Read the model definition and answer for the solid it produces. Units are mm, in the model's axes. A direction names the side the tool comes from. Coordinates: 2 decimals unless noted, no trailing zeros. Write each loop counter-clockwise with the first axis right and the second up, starting at its lowest first coordinate (ties: lowest second). Pieces come first, ordered by that corner, then holes. Notation, with made-up numbers: (87, 74) - (128, 74) arc R22 cw to (128, 113) - close; hole circle Ø11 at (-28, 5.5). An arc over 180 degrees is marked (long way). Return JSON: item names as keys, results as strings.
```python
from build123d import *

# Parameters (mm, degrees)
F0_R            = 5
F1_DEPTH        = 50
F2_R            = 15
F3_DEPTH        = 5
F3_COPIES_COUNT = 3
F4_W            = 25
F4_H            = 25
F5_DEPTH        = 5
F5_COPIES_COUNT = 3
F7_DEPTH        = 5
F7_COPIES_COUNT = 3


# Not quite as in the source:
# - a pattern or mirror of a feature is missing from the dataset's text; its kind, count and spacing are read off the source's solid


with BuildPart() as f1:
    # F0 (on Top) → F1 (new body)
    with BuildSketch(Plane.XY):
        Polygon((64.2787609687, 76.6044443119), (0, 100), (-64.2787609687, 76.6044443119), (-98.4807753012, 17.3648177667), (-86.6025403784, -50), (-34.2020143326, -93.9692620786), (34.2020143326, -93.9692620786), (86.6025403784, -50), (98.4807753012, 17.3648177667), align=None)
        Circle(F0_R, mode=Mode.SUBTRACT)
    extrude(amount=F1_DEPTH)

    # F2 (on face) → F3 (cut)
    with BuildSketch(Plane(origin=(60.4022773555, -71.9846310393, 0), x_dir=(0.7660444431, 0.6427876097, 0), z_dir=(0.6427876097, -0.7660444431, 0))):
        with Locations((0, 25)):
            Circle(F2_R)
    f3 = extrude(amount=-F3_DEPTH, mode=Mode.SUBTRACT)

    # F3_copies: F3 ×3 about axis
    f3_copies_axis = Axis((0, 0, 0), (0, 0, 1))
    for i in range(1, F3_COPIES_COUNT):
        add(f3.rotate(f3_copies_axis, i * 360 / F3_COPIES_COUNT), mode=Mode.SUBTRACT)

    # F4 (on face) → F5 (cut)
    with BuildSketch(Plane(origin=(-60.4022773555, -71.9846310393, 0), x_dir=(0.7660444431, -0.6427876097, 0), z_dir=(-0.6427876097, -0.7660444431, 0))):
        with Locations((0, 25)):
            Rectangle(F4_W, F4_H)
    f5 = extrude(amount=-F5_DEPTH, mode=Mode.SUBTRACT)

    # F5_copies: F5 ×3 about axis
    f5_copies_axis = Axis((0, 0, 0), (0, 0, 1))
    for i in range(1, F5_COPIES_COUNT):
        add(f5.rotate(f5_copies_axis, i * 360 / F5_COPIES_COUNT), mode=Mode.SUBTRACT)

    # F6 (on face) → F7 (cut)
    with BuildSketch(Plane.XZ.offset(93.9692620786)):
        Polygon((-8.25, 10.7105808376), (16.5, 25), (-8.25, 39.2894191624), align=None)
    f7 = extrude(amount=-F7_DEPTH, mode=Mode.SUBTRACT)

    # F7_copies: F7 ×3 about axis
    f7_copies_axis = Axis((0, 0, 0), (0, 0, 1))
    for i in range(1, F7_COPIES_COUNT):
        add(f7.rotate(f7_copies_axis, i * 360 / F7_COPIES_COUNT), mode=Mode.SUBTRACT)


solid = f1.part
```
(1) Determine the mould class of faces 4 (the face through (7, -93.969, 19)), 5 (the face through (48.391, -82.063, 24.65)), 6 (the face through (92.28, -3.58, 24.83)) for opening direction X: +X half, -X half, draft (parallel to the pull), parting line (faces both ways), or undercut.
Answer:
{"face 4": "draft", "face 5": "+X half", "face 6": "undercut"}
(2) A cutting plane is placed at A-A (z = 44.5). Determine the outline of the cut face in (x, y), and give its area (3 significant figures).
Answer:
{"outline": "(-98.48, 17.36) - (-86.6, -50) - (-34.2, -93.97) - (34.2, -93.97) - (86.6, -50) - (98.48, 17.36) - (64.28, 76.6) - (0, 100) - (-64.28, 76.6) - close; hole circle Ø10 at (0, 0)", "area": "28,800 mm²"}
(3) Straight lines are drawn through the part: line 1 (Y direction, x = 0, z = 34); line 2 (Y direction, x = 0, z = 37); line 3 (Z direction, x = -21, y = 90). For each, find the intervals that lie inside material, in ascending order. Write a range as from..to.
Answer:
{"line 1": "-88.97..-5, 5..100", "line 2": "-93.97..-5, 5..100", "line 3": "0..12.5, 37.5..50"}
(4) Which of the six approach directions +Z, -Z, +X, -X, +Y, -Y give full straight-line access (tool end or side, diameter ignored) to faces 1 (the face through (1, -88.969, 25)), 2 (the face through (-43.042, 81.711, 24.825)), 3 (the face through (57.027, -68.289, 25.21))?
Answer:
{"face 1": "-Y", "face 2": "+Y", "face 3": "none"}
(5) Flat-ended cylindrical pins translate along their axes: P1, Ø3, axis at x = 11, z = 22.5, coming from the +Y side; P2, Ø9, axis at x = 0, y = 0, coming from the -Z side; P3, Ø3, axis at y = -18, z = 9, coming from the +X side; P4, Ø12, axis at y = -17, z = 16, coming from the +X side. Find the tip coordinate at first contact, or state that the pin passes through.
Answer:
{"P1": "y = 96.54", "P2": "through", "P3": "x = 92.51", "P4": "x = 93.28"}
(6) A cutting plane is placed at B-B (x = -60). Determine the outline of the cut face in (y, z), and give its area (3 significant figures).
Answer:
{"outline": "(-72.32, 0) - (78.16, 0) - (78.16, 50) - (-72.32, 50) - (-72.32, 37.5) - (-65.8, 37.5) - (-65.8, 12.5) - (-72.32, 12.5) - close", "area": "7,360 mm²"}
